Geometry check sheet. Reference: the model listing, model coordinates, mm. Face numbers are marked on the shaded views. Round coordinates to 2 decimals unless told otherwise and drop trailing zeros. Write each loop counter-clockwise with the first axis right and the second up, starting at its lowest first coordinate (ties: lowest second). Pieces come first, ordered by that corner, then holes. Notation, with made-up numbers: M 16,-32 L 41,-32 A22 ccw 41,-10 Z; hole C -30.75,45.25 d3. An arc over 180 degrees is marked long. One line per item, written item: value. Start each with the question number.
1. Section check C-C (y = 0.55). Record the boundary of the cut face in (x, z), and give its area (3 significant figures).
2. Release check for a two-part mould opening along X. For the marked faces 1, 2 and 3 record: pulls with the +X half, pulls with the -X half, needs draft (parallel to the pull), parting line crosses it, or undercut.
3. Scan lines: probe 1 along X at (y, z) = (0.65, 0); probe 2 along X at (y, z) = (1.1, -1.25); probe 3 along Z at (x, y) = (-3.75, 1.15). Record each from-to range of solid material in increasing order. Write a range as [from, to].
4. Depth check by flat-ended pin: P1, Ø4, axis at x = 0, z = 0, coming from the -Y side; P2, Ø1.9, axis at x = -3, z = 0, coming from the +Y side. Enter the tip coordinate at first touch or a pass-through.
5. Section check A-A (x = -3). Record the boundary of the cut face in (y, z), and give its area (3 significant figures).
6. Section check B-B (z = 0). Record the boundary of the cut face in (x, y), and give its area (3 significant figures).
7. Section check D-D (z = 1.25). Record the boundary of the cut face in (x, y), and give its area (3 significant figures).
from build123d import *

# Parameters (mm, degrees)
SKETCH1_W           = 12
SKETCH1_H           = 7
BOSS_EXTRUDE1_DEPTH = 2
SKETCH2_R           = 1.6
CUT_EXTRUDE1_DEPTH  = 8.228416147
FILLET1_R           = 0.8


with BuildPart() as part:
    # Sketch1 → Boss-Extrude1 (new body)
    with BuildSketch(Plane(origin=(0, 0, 0), x_dir=(1, 0, 0), z_dir=(0, 1, 0))):
        Rectangle(SKETCH1_W, SKETCH1_H)
    extrude(amount=BOSS_EXTRUDE1_DEPTH)

    # Sketch2 → Cut-Extrude1 (cut, through all)
    with BuildSketch(Plane(origin=(0, 2, 0), x_dir=(1, 0, 0), z_dir=(0, 1, 0))):
        with Locations(Location((-3, 0, 0), (0, 0, 270))):
            Circle(SKETCH2_R)
        with Locations(Location((3, 0, 0), (0, 0, 270))):
            Circle(SKETCH2_R)
    extrude(amount=-CUT_EXTRUDE1_DEPTH, mode=Mode.SUBTRACT)

    # Fillet1
    fillet1_edges = [part.edges().sort_by_distance(p)[0] for p in [
        (6, 1, 3.5),
        (-6, 1, 3.5),
        (-6, 1, -3.5),
        (6, 1, -3.5),
    ]]
    fillet(fillet1_edges, radius=FILLET1_R)


solid = part.part
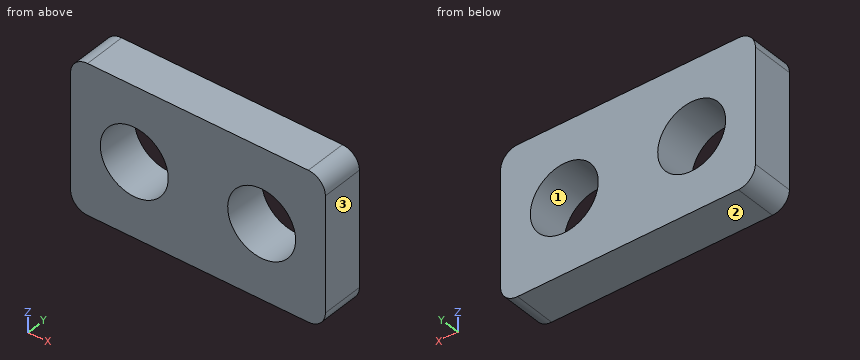
Result sheet:
1. outline: M -6,-2.7 A0.8 ccw -5.2,-3.5 L 5.2,-3.5 A0.8 ccw 6,-2.7 L 6,2.7 A0.8 ccw 5.2,3.5 L -5.2,3.5 A0.8 ccw -6,2.7 Z; hole C -3,0 d3.2; hole C 3,0 d3.2
1. area: 67.4 mm2
2. face 1: undercut
2. face 2: needs draft
2. face 3: pulls with the +X half
3. probe 1: x = [-6, -4.6], [-1.4, 1.4], [4.6, 6]
3. probe 2: x = [-6, -4], [-2, 2], [4, 6]
3. probe 3: z = [-3.5, -1.41], [1.41, 3.5]
4. P1: stops at y = 0
4. P2: passes through
5. outline: M 0,-3.5 L 2,-3.5 L 2,-1.6 L 0,-1.6 Z; M 0,1.6 L 2,1.6 L 2,3.5 L 0,3.5 Z
5. area: 7.60 mm2
6. outline: M -6,0 L -4.6,0 L -4.6,2 L -6,2 Z; M -1.4,0 L 1.4,0 L 1.4,2 L -1.4,2 Z; M 4.6,0 L 6,0 L 6,2 L 4.6,2 Z
6. area: 11.2 mm2
7. outline: M -6,0 L -4,0 L -4,2 L -6,2 Z; M -2,0 L 2,0 L 2,2 L -2,2 Z; M 4,0 L 6,0 L 6,2 L 4,2 Z
7. area: 16.0 mm2
